Here's how the part is built. I have some questions about the finished solid (model axes, mm). Round coordinates to 2 decimals unless told otherwise and drop trailing zeros. Order: outer loops, then holes, each group sorted by start corner. A loop starts at its lowest first (then second) coordinate and runs counter-clockwise, first axis right, second up. Notation, with made-up numbers: (-39.75, 81.25) - (-12.75, 81.25) arc R21 ccw to (-12.75, 91.25) - close; hole circle Ø11 at (6, 57). An arc over 180 degrees is marked (long way). One line per item, written item: value.
from build123d import *

# Parameters (mm, degrees)
SKETCH1_R           = 80
BOSS_EXTRUDE1_DEPTH = 5


with BuildPart() as part:
    # Sketch1 → Boss-Extrude1 (new body)
    with BuildSketch(Plane.XY):
        Polygon((-110, 120), (-120, 120), (-120, 110), (-125, 110), (-125, 80), (-120, 80), (-120, 15), (-125, 15), (-125, -15), (-120, -15), (-120, -80), (-125, -80), (-125, -110), (-120, -110), (-120, -120), (-110, -120), (-110, -125), (-80, -125), (-80, -120), (-15, -120), (-15, -125), (15, -125), (15, -120), (80, -120), (80, -125), (110, -125), (110, -120), (120, -120), (120, -110), (125, -110), (125, -80), (120, -80), (120, -15), (125, -15), (125, 15), (120, 15), (120, 80), (125, 80), (125, 110), (120, 110), (120, 120), (110, 120), (110, 125), (80, 125), (80, 120), (15, 120), (15, 125), (-15, 125), (-15, 120), (-80, 120), (-80, 125), (-110, 125), align=None)
        Circle(SKETCH1_R, mode=Mode.SUBTRACT)
    extrude(amount=BOSS_EXTRUDE1_DEPTH)


solid = part.part
Q1. If we section it at A-A, the plane y = 0: Please give me the cut outline in (x, z), then the cut area to 3 significant figures.
Results list:
outline: (-125, 0) - (-80, 0) - (-80, 5) - (-125, 5) - close; (80, 0) - (125, 0) - (125, 5) - (80, 5) - close
area: 450 mm²
Q2. If I drill on line 1 along Y through (x, z) = (0, 2.6); line 2 along X through (y, z) = (30, 1.8), over which ranges is the centre line in solid material (lowest first)?
Results list:
line 1: -125 to -80, 80 to 125
line 2: -120 to -74.16, 74.16 to 120
Q3. We'd pull the mould along Y, two halves only. Please class faces 1 (the cylindrical face through (-17.34, -78.1, 2.46)), 2 (the flat face through (-57, 57, 0)): released by +Y, released by -Y, zero draft, split by the parting line, or undercut.
Results list:
face 1: undercut
face 2: zero draft
Q4. Will these pins go through, and if not, where does the flat tip stop? pin 1 (1.5 mm diameter, centred on y = 41.5, z = 1.5, fed in from +X); pin 2 (1.5 mm diameter, centred on x = 122.5, z = 2, fed in from -Y); pin 3 (1.5 mm diameter, centred on y = -121.5, z = 2.5, fed in from -X); pin 4 (1.5 mm diameter, centred on x = 47.5, y = 98, fed in from -Z).
Results list:
pin 1: x = 120
pin 2: y = -110
pin 3: x = -110
pin 4: z = 0
